from build123d import *

# Parameters (mm, degrees)
SKETCH1_W           = 300
SKETCH1_H           = 150
SKETCH1_R           = 14.235
BOSS_EXTRUDE1_DEPTH = 3
CUT_EXTRUDE1_REACH  = 5
SKETCH2_R           = 3.225
SKETCH3_R           = 2.75
CUT_EXTRUDE2_DEPTH  = 4
CUT_EXTRUDE3_DEPTH  = 4
CUT_EXTRUDE4_DEPTH  = 10
CUT_EXTRUDE5_DEPTH  = 10
SKETCH7_R           = 2.75
CUT_EXTRUDE6_DEPTH  = 4


with BuildPart() as part:
    # Sketch1 → Boss-Extrude1 (new body)
    with BuildSketch(Plane(origin=(0, 0, 0), x_dir=(0, 0, -1), z_dir=(1, 0, 0))):
        with Locations((150, 75)):
            Rectangle(SKETCH1_W, SKETCH1_H)
        with Locations((30, 55)):
            Circle(SKETCH1_R, mode=Mode.SUBTRACT)
    extrude(amount=BOSS_EXTRUDE1_DEPTH)

    # Sketch2 → Cut-Extrude1 (cut, up to next)
    with BuildSketch(Plane.ZY, mode=Mode.PRIVATE) as cut_extrude1_sk1:
        with Locations((-290, 140)):
            Circle(SKETCH2_R)
    cut_extrude1_tool1 = extrude(cut_extrude1_sk1.sketch, amount=-CUT_EXTRUDE1_REACH, mode=Mode.PRIVATE) & part.part
    add(cut_extrude1_tool1.solids().sort_by_distance((0, 140, -290))[0], mode=Mode.SUBTRACT)
    # Sketch2 → Cut-Extrude1 (cut, up to next)
    with BuildSketch(Plane.ZY, mode=Mode.PRIVATE) as cut_extrude1_sk2:
        with Locations((-10, 110)):
            Circle(SKETCH2_R)
    cut_extrude1_tool2 = extrude(cut_extrude1_sk2.sketch, amount=-CUT_EXTRUDE1_REACH, mode=Mode.PRIVATE) & part.part
    add(cut_extrude1_tool2.solids().sort_by_distance((0, 110, -10))[0], mode=Mode.SUBTRACT)
    # Sketch2 → Cut-Extrude1 (cut, up to next)
    with BuildSketch(Plane.ZY, mode=Mode.PRIVATE) as cut_extrude1_sk3:
        with Locations((-290, 30)):
            Circle(SKETCH2_R)
    cut_extrude1_tool3 = extrude(cut_extrude1_sk3.sketch, amount=-CUT_EXTRUDE1_REACH, mode=Mode.PRIVATE) & part.part
    add(cut_extrude1_tool3.solids().sort_by_distance((0, 30, -290))[0], mode=Mode.SUBTRACT)
    # Sketch2 → Cut-Extrude1 (cut, up to next)
    with BuildSketch(Plane.ZY, mode=Mode.PRIVATE) as cut_extrude1_sk4:
        with BuildLine():
            Line((-185.611446384, 98.478413591), (-225.611446384, 98.478413591))
            ThreePointArc((-225.611446384, 98.478413591), (-228.841446384, 101.708413591), (-225.611446384, 104.938413591))
            Line((-225.611446384, 104.938413591), (-185.611446384, 104.938413591))
            ThreePointArc((-185.611446384, 104.938413591), (-182.381446384, 101.708413591), (-185.611446384, 98.478413591))
        make_face()
    cut_extrude1_tool4 = extrude(cut_extrude1_sk4.sketch, amount=-CUT_EXTRUDE1_REACH, mode=Mode.PRIVATE) & part.part
    add(cut_extrude1_tool4.solids().sort_by_distance((0, 101.708414, -205.611446))[0], mode=Mode.SUBTRACT)
    # Sketch2 → Cut-Extrude1 (cut, up to next)
    with BuildSketch(Plane.ZY, mode=Mode.PRIVATE) as cut_extrude1_sk5:
        with BuildLine():
            Line((-233.743605698, 22.681694356), (-193.743605698, 22.681694356))
            ThreePointArc((-193.743605698, 22.681694356), (-190.518605698, 19.456694356), (-193.743605698, 16.231694356))
            Line((-193.743605698, 16.231694356), (-233.743605698, 16.231694356))
            ThreePointArc((-233.743605698, 16.231694356), (-236.968605698, 19.456694356), (-233.743605698, 22.681694356))
        make_face()
    cut_extrude1_tool5 = extrude(cut_extrude1_sk5.sketch, amount=-CUT_EXTRUDE1_REACH, mode=Mode.PRIVATE) & part.part
    add(cut_extrude1_tool5.solids().sort_by_distance((0, 19.456694, -213.743606))[0], mode=Mode.SUBTRACT)

    # Sketch3 → Cut-Extrude2 (cut, through all)
    with BuildSketch(Plane(origin=(3, 0, 0), x_dir=(0, 0, -1), z_dir=(1, 0, 0))):
        with Locations((14.005743185, 74.73179538)):
            Circle(SKETCH3_R)
        with Locations((45.994256815, 35.26820462)):
            Circle(SKETCH3_R)
    extrude(amount=-CUT_EXTRUDE2_DEPTH, mode=Mode.SUBTRACT)

    # Sketch4 → Cut-Extrude3 (cut, through all)
    with BuildSketch(Plane(origin=(3, 0, 0), x_dir=(0, 0, -1), z_dir=(1, 0, 0))):
        Polygon((71, 9), (0, 35), (0, 0), (71, 0), align=None)
    extrude(amount=-CUT_EXTRUDE3_DEPTH, mode=Mode.SUBTRACT)

    # Sketch5 → Cut-Extrude4 (cut)
    with BuildSketch(Plane(origin=(3, 0, 0), x_dir=(0, 0, -1), z_dir=(1, 0, 0))):
        Polygon((228.92403237, 9), (250.717958721, 16.875947155), (250.717958721, 150), (312.660420977, 150), (312.660420977, -2.829604392), (228.92403237, 0), align=None)
    extrude(amount=-CUT_EXTRUDE4_DEPTH, mode=Mode.SUBTRACT)

    # Sketch6 → Cut-Extrude5 (cut)
    with BuildSketch(Plane(origin=(3, 0, 0), x_dir=(0, 0, -1), z_dir=(1, 0, 0))):
        Polygon((0, 85.848631797), (186.802640374, 119.641480316), (250.717958721, 119.641480316), (250.717958721, 150), (0, 150), align=None)
    extrude(amount=-CUT_EXTRUDE5_DEPTH, mode=Mode.SUBTRACT)

    # Sketch7 → Cut-Extrude6 (cut, through all)
    with BuildSketch(Plane.ZY):
        with Locations((-209.962016185, 5)):
            Circle(SKETCH7_R)
        with Locations((-149.962016185, 5)):
            Circle(SKETCH7_R)
        with Locations((-89.962016185, 5)):
            Circle(SKETCH7_R)
    extrude(amount=-CUT_EXTRUDE6_DEPTH, mode=Mode.SUBTRACT)


solid = part.part
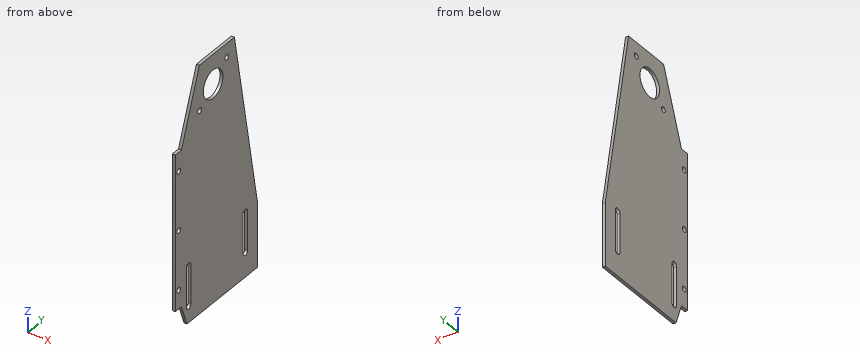
For this review, take the finished solid that the model builds, in its own axes (mm). Round coordinates to 2 decimals unless told otherwise and drop trailing zeros. Write each loop counter-clockwise with the first axis right and the second up, starting at its lowest first coordinate (ties: lowest second). Pieces come first, ordered by that corner, then holes. Notation, with made-up numbers: (-9.5, 50) - (6.5, 50) arc R30 cw to (6.5, 86) - close; hole circle Ø7 at (34.5, 78.25). An arc over 180 degrees is marked (long way). Use a Markdown table: item, result.
Q1. Clearance check with flat-ended pins moving along their axes: pin 1 (0.9 mm diameter, centred on x = 1, y = 3, fed in from +Z); pin 2 (3.5 mm diameter, centred on y = 35.27, z = -45.99, fed in from +X); pin 3 (1.5 mm diameter, centred on x = 2, z = -43, fed in from +Y). State where each tip first meets the part, or that it passes through.
Derived:
| item | result |
|---|---|
| pin 1 | stops at z = -71 |
| pin 2 | passes through |
| pin 3 | stops at y = 93.76 |
Q2. We need section B-B (y = 55). Give the boundary of the cut face in (x, z) (3 decimals).
Derived:
| item | result |
|---|---|
| outline | (0, -250.718) - (3, -250.718) - (3, -44.235) - (0, -44.235) - close; (0, -15.765) - (3, -15.765) - (3, 0) - (0, 0) - close |
Q3. Wall thickness on line 1 along Y through (x, z) = (0.65, -200); line 2 along Z through (x, y) = (1.6, 54.5); line 3 along Z through (x, y) = (2.45, 63.5): over which ranges is each line inside the solid? List them lowest first.
Derived:
| item | result |
|---|---|
| line 1 | y = 0 to 16.23, 22.68 to 98.48, 104.94 to 119.64 |
| line 2 | z = -250.72 to -44.23, -15.77 to 0 |
| line 3 | z = -250.72 to -41.42, -18.58 to 0 |
Q4. We need section A-A (y = 5). Give the boundary of the cut face in (x, z).
Derived:
| item | result |
|---|---|
| outline | (0, -228.92) - (3, -228.92) - (3, -212.71) - (0, -212.71) - close; (0, -207.21) - (3, -207.21) - (3, -152.71) - (0, -152.71) - close; (0, -147.21) - (3, -147.21) - (3, -92.71) - (0, -92.71) - close; (0, -87.21) - (3, -87.21) - (3, -71) - (0, -71) - close |
Q5. We need section C-C (z = -33.5). Give the boundary of the cut face in (x, y).
Derived:
| item | result |
|---|---|
| outline | (0, 22.73) - (3, 22.73) - (3, 41.2) - (0, 41.2) - close; (0, 68.8) - (3, 68.8) - (3, 91.91) - (0, 91.91) - close |
Q6. We need section D-D (x = 2.15). State how many separate pieces and enclosed holes the cut face has, plus the area to 3 significant figures.
Derived:
| item | result |
|---|---|
| separate pieces | 1 |
| enclosed holes | 8 |
| area | 23,700 mm2 |
